from build123d import *

# Parameters (mm, degrees)
SKETCH_1_R          = 1.6
EXTRUDE_1_DEPTH     = 25
SKETCH_2_W          = 2.5
SKETCH_2_H          = 19.896013553
EXTRUDE_2_DEPTH     = 40
SKETCH_3_R          = 1.5
CUT_EXTRUDE_1_DEPTH = 90.582364336
SKETCH_4_W          = 40
SKETCH_4_H          = 4
EXTRUDE_3_DEPTH     = 25
FILLET_4_R          = 10
FILLET_5_R          = 10


with BuildPart() as part:
    # 草图1 → 凸台-拉伸1 (new body)
    # profile 1 of 2: a face of its own
    with BuildSketch(Plane(origin=(0, 0, 0), x_dir=(0, 0, -1), z_dir=(1, 0, 0))):
        with BuildLine():
            ThreePointArc((-47.85, 0), (-46.25, 1.6), (-44.65, 0))
            Line((-44.65, 0), (-42.5, 0))
            ThreePointArc((-42.5, 0), (-16.298006013, 39.25079617), (30, 30.103986447))
            Line((30, 30.103986447), (30, 50))
            Line((30, 50), (0, 50))
            ThreePointArc((0, 50), (-35.355339059, 35.355339059), (-50, 0))
            Line((-50, 0), (-47.85, 0))
        make_face()
        with Locations((-23.125, 40.053674925)):
            Circle(SKETCH_1_R, mode=Mode.SUBTRACT)
        with Locations((23.125, 40.053674925)):
            Circle(SKETCH_1_R, mode=Mode.SUBTRACT)
    # profile 2 of 2: a face of its own
    with BuildSketch(Plane(origin=(0, 0, 0), x_dir=(0, 0, -1), z_dir=(1, 0, 0))):
        with BuildLine():
            Line((-42.5, 0), (-44.65, 0))
            ThreePointArc((-44.65, 0), (-46.25, -1.6), (-47.85, 0))
            Line((-47.85, 0), (-50, 0))
            ThreePointArc((-50, 0), (-35.355339059, -35.355339059), (0, -50))
            Line((0, -50), (30, -50))
            Line((30, -50), (30, -30.103986447))
            ThreePointArc((30, -30.103986447), (-16.298006013, -39.25079617), (-42.5, 0))
        make_face()
        with Locations((-23.125, -40.053674925)):
            Circle(SKETCH_1_R, mode=Mode.SUBTRACT)
        with Locations((23.125, -40.053674925)):
            Circle(SKETCH_1_R, mode=Mode.SUBTRACT)
    extrude(amount=EXTRUDE_1_DEPTH)

    # 草图2 → 凸台-拉伸2 (add)
    with BuildSketch(Plane(origin=(0, 0, -30), x_dir=(-1, 0, 0), z_dir=(0, 0, -1))):
        with Locations((-23.75, 40.051993223)):
            Rectangle(SKETCH_2_W, SKETCH_2_H)
        with Locations((-1.25, 40.051993223)):
            Rectangle(SKETCH_2_W, SKETCH_2_H)
        with Locations((-1.25, -40.051993223)):
            Rectangle(SKETCH_2_W, SKETCH_2_H)
        with Locations((-23.75, -40.051993223)):
            Rectangle(SKETCH_2_W, SKETCH_2_H)
    extrude(amount=EXTRUDE_2_DEPTH)

    # 草图3 → 切除-拉伸1 (cut, through all)
    with BuildSketch(Plane(origin=(25, 0, 0), x_dir=(0, 0, -1), z_dir=(1, 0, 0))):
        with Locations((60, -40.051993223)):
            Circle(SKETCH_3_R)
        with Locations((40, -40.051993223)):
            Circle(SKETCH_3_R)
        with Locations(Location((40.013969678, 40.055824633, 0), (0, 0, 270))):
            Circle(SKETCH_3_R)
        with Locations(Location((60.013968461, 40.048849195, 0), (0, 0, 270))):
            Circle(SKETCH_3_R)
    extrude(amount=-CUT_EXTRUDE_1_DEPTH, mode=Mode.SUBTRACT)

    # 草图4 → 凸台-拉伸3 (add)
    with BuildSketch(Plane(origin=(25, 0, 0), x_dir=(0, 0, -1), z_dir=(1, 0, 0))):
        with Locations((20, 52)):
            Rectangle(SKETCH_4_W, SKETCH_4_H)
        with Locations((20, -52)):
            Rectangle(SKETCH_4_W, SKETCH_4_H)
    extrude(amount=-EXTRUDE_3_DEPTH)

    # 圆角4
    # the kernel refuses this fillet: 10 mm, written as the material it takes off along each edge
    with BuildSketch(Plane(origin=(45, -54, 0), x_dir=(0, 0, -1), z_dir=(-1, 0, 0))) as fillet_4_piece_1:
        with BuildLine():
            CenterArc((8, -10), FILLET_4_R, 90, 53.130102354)
            Line((0, -4), (-0.16, -3.88))
            ThreePointArc((-0.16, -3.88), (-0.2, -2), (-0.2, 0))
            Line((-0.2, 0), (0, 0.2))
            Line((0, 0.2), (8, 0.2))
            Line((8, 0.2), (8, 0))
        make_face()
    extrude(amount=65, mode=Mode.SUBTRACT)
    with BuildSketch(Plane(origin=(45, 54, 0), x_dir=(0, 0, -1), z_dir=(-1, 0, 0))) as fillet_4_piece_2:
        with BuildLine():
            CenterArc((8, 10), FILLET_4_R, 216.869897646, 53.130102354)
            Line((0, 4), (-0.16, 3.88))
            ThreePointArc((-0.16, 3.88), (-0.2, 2), (-0.2, 0))
            Line((-0.2, 0), (0, -0.2))
            Line((0, -0.2), (8, -0.2))
            Line((8, -0.2), (8, 0))
        make_face()
    extrude(amount=65, mode=Mode.SUBTRACT)

    # 圆角5
    fillet_5_edges = [part.edges().sort_by_distance(p)[0] for p in [
        (12.5, -50, 0),
        (12.5, 50, 0),
    ]]
    fillet(fillet_5_edges, radius=FILLET_5_R)


solid = part.part
Geometry: final body of the model. Coordinates: model frame, mm. A direction names the side the tool comes from. Give positions to 0.01 mm unless a question says otherwise; leave off trailing zeros. Loops run counter-clockwise (first coordinate to the right, second up) from the corner with the lowest first, then second, coordinate; pieces in that order, holes last. Notation, with made-up numbers: M 39,-15 L 84,-15 A14 cw 84,-5 Z; hole C 10,27 d2. An arc over 180 degrees is marked long. Put each result on its own line as item: value. Start each with the question number.
1) Cut plane B-B (y = 47.5). Output: boundary loops of the cut face in (x, z).
2) Access query for faces 4 (the flat face through (1, -50, -55)), 5 (the flat face through (1, 50, -55)), 6 (the flat face through (13, -50, -35)). Directions: +Z, -Z, +X, -X, +Y, -Y. A direction counts if a zero-diameter tool reaches every point of the face in a straight line with its end or side. Return the directions, or none.
3) Cut plane A-A (z = 46.25). Output: boundary loops of the cut face in (x, y).
4) Ray query, line 1 along X through (y, z) = (47, -42.5); line 2 along Y through (x, z) = (23.25, -22.5); line 3 along Y through (x, z) = (21.75, -38.5). Return the intervals inside material, ascending.
5) Cut plane D-D (y = -45). Output: boundary loops of the cut face in (x, z), then the cut area to 3 significant figures.
6) Contact query for flat-ended pins moving along their axis: pin 1 (2 mm diameter, centred on x = 23.5, z = -43.5, fed in from +Y); pin 2 (5 mm diameter, centred on x = 13.5, z = -3.5, fed in from +Y); pin 3 (10 mm diameter, centred on x = 21.5, z = -2.5, fed in from +Y). Output: stop coordinate, or through.
7) Pull-direction query (X, two-part tool) for faces 1 (the flat face through (12, -40, -30)), 2 (the cylindrical face through (1.267, -40.627, -61.386)), 3 (the flat face through (22.5, 40, -50)); classes: pulls with the +X half, pulls with the -X half, needs draft (parallel to the pull), parting line crosses it, or undercut.
8) Cut plane C-C (x = 4.5). Give the number of separate pieces and of enclosed holes in the cut face, then the cut area to 3 significant figures.
Verdict:
1. outline: M 0,-70 L 2.5,-70 L 2.5,-30 L 22.5,-30 L 22.5,-70 L 25,-70 L 25,15.61 L 0,15.61 Z
2. face 4: -Z, +X, -X, -Y
2. face 5: -Z, +X, -X, +Y
2. face 6: -Z
3. outline: M 0,-19 L 25,-19 L 25,-1.6 L 0,-1.6 Z; M 0,1.6 L 25,1.6 L 25,19 L 0,19 Z
4. line 1: 0 to 2.5, 22.5 to 25
4. line 2: -54 to -41.53, -38.58 to -36.06, 36.06 to 38.58, 41.53 to 54
4. line 3: -54 to -50, 50 to 54
5. outline: M 0,-70 L 2.5,-70 L 2.5,-30 L 22.5,-30 L 22.5,-70 L 25,-70 L 25,21.79 L 0,21.79 Z
5. area: 1,490 mm2
6. pin 1: y = 50
6. pin 2: y = 53.8
6. pin 3: y = 53.99
7. face 1: undercut
7. face 2: needs draft
7. face 3: undercut
8. separate pieces: 1
8. enclosed holes: 5
8. area: 2,030 mm2
